from build123d import *

# Parameters (mm, degrees)
F1_DEPTH  = 25.4
F3_DEPTH  = 12.7
F4_R      = 19.05
F5_R      = 19.05
F6_R      = 20
F7_DEPTH  = 12.7
F8_R      = 21.5
F9_DEPTH  = 4.6
F10_R     = 33
F10_R_2   = 26.5
F11_DEPTH = 4
F12_W     = 3.69096
F12_H     = 9.525
F13_DEPTH = 8.7


with BuildPart() as f1:
    # F0 (on Top) → F1 (new body)
    with BuildSketch(Plane.XY):
        Polygon((22.73028, 39.37), (-22.73028, 39.37), (-45.46056, 0), (-22.73028, -39.37), (22.73028, -39.37), (45.46056, 0), align=None)
    extrude(amount=F1_DEPTH)

    # F2 (on face) → F3 (cut)
    with BuildSketch(Plane.XY.offset(25.4)):
        Polygon((21.26381, 36.83), (-21.26381, 36.83), (-42.527621, 0), (-21.26381, -36.83), (21.26381, -36.83), (42.527621, 0), align=None)
    extrude(amount=-F3_DEPTH, mode=Mode.SUBTRACT)

    # F4
    f4_edges = [f1.edges().sort_by_distance(p)[0] for p in [
        (21.26381, 36.83, 19.05),
        (-21.26381, 36.83, 19.05),
        (-42.527621, 0, 19.05),
        (42.527621, 0, 19.05),
        (21.26381, -36.83, 19.05),
        (-21.26381, -36.83, 19.05),
    ]]
    fillet(f4_edges, radius=F4_R)

    # F5
    f5_edges = [f1.edges().sort_by_distance(p)[0] for p in [
        (-22.73028, -39.37, 12.7),
        (22.73028, -39.37, 12.7),
        (45.46056, 0, 12.7),
        (-45.46056, 0, 12.7),
        (-22.73028, 39.37, 12.7),
        (22.73028, 39.37, 12.7),
    ]]
    fillet(f5_edges, radius=F5_R)

    # F6 (on face) → F7 (cut, through all)
    with BuildSketch(Plane(origin=(0, 0, 0), x_dir=(1, 0, 0), z_dir=(0, 0, -1))):
        Circle(F6_R)
    extrude(amount=-F7_DEPTH, mode=Mode.SUBTRACT)

    # F8 (on face) → F9 (cut)
    with BuildSketch(Plane(origin=(0, 0, 0), x_dir=(1, 0, 0), z_dir=(0, 0, -1))):
        Circle(F8_R)
    extrude(amount=-F9_DEPTH, mode=Mode.SUBTRACT)

    # F10 (on face) → F11 (cut)
    with BuildSketch(Plane(origin=(0, 0, 0), x_dir=(1, 0, 0), z_dir=(0, 0, -1))):
        Circle(F10_R)
        Circle(F10_R_2, mode=Mode.SUBTRACT)
    extrude(amount=-F11_DEPTH, mode=Mode.SUBTRACT)

    # F12 (on face) → F13 (cut, through all)
    with BuildSketch(Plane(origin=(0, 0, 4), x_dir=(1, 0, 0), z_dir=(0, 0, -1))):
        with Locations((29.75, 4.7625)):
            Rectangle(F12_W, F12_H)
        with Locations((29.75, -4.7625)):
            Rectangle(F12_W, F12_H)
    extrude(amount=-F13_DEPTH, mode=Mode.SUBTRACT)


solid = f1.part
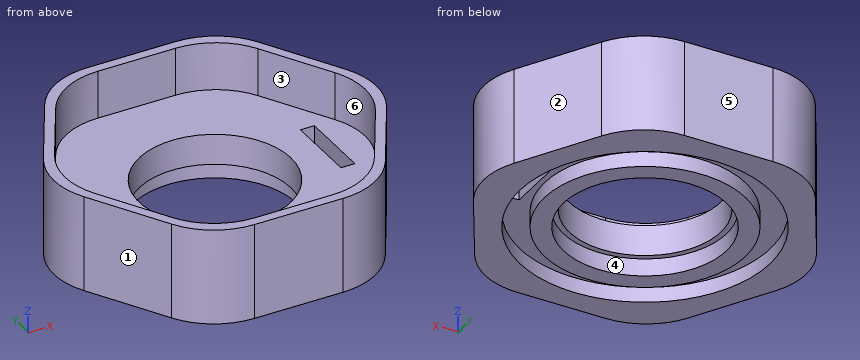
Read the model definition and answer for the solid it produces. Units are mm, in the model's axes. Face numbers are marked on the shaded views. A direction names the side the tool comes from. Coordinates: 2 decimals unless noted, no trailing zeros. Loops run counter-clockwise (first coordinate to the right, second up) from the corner with the lowest first, then second, coordinate; pieces in that order, holes last. Notation, with made-up numbers: (-2, 8) -> (50, 8) arc R9 cw to (50, 16) -> close; hole circle Ø2 at (57, -21). An arc over 180 degrees is marked (long way). Answer in a Markdown table with one row per item.
Item 1: For the marked faces 4, 5 and 6, determine the directions among +Z, -Z, +X, -X, +Y, -Y from which every point of the face is accessible in a straight line to the end or side of a thin tool.
Returned:
| item | result |
|---|---|
| face 4 | -Z |
| face 5 | +Z, -Z, +X, -X, +Y |
| face 6 | +Z |
Item 2: Each of these flat-tipped pins is pushed along its axis until it touches: P1, Ø7, axis at y = -2.5, z = 7, coming from the -X side; P2, Ø1.1, axis at x = 29.5, z = 7, coming from the -Y side; P3, Ø1.5, axis at x = -26.5, y = 31.5, coming from the -Z side; P4, Ø12, axis at x = -26.5, z = 14.5, coming from the -Y side. Where does it stop, or does it pass through?
Returned:
| item | result |
|---|---|
| P1 | stops at x = -42.51 |
| P2 | stops at y = -28.6 |
| P3 | stops at z = 0 |
| P4 | stops at y = -37.23 |
Item 3: A cutting plane is placed at D-D on y = 8.5. Determine the outline of the cut face in (x, z), plus the area to 3 significant figures.
Returned:
| item | result |
|---|---|
| outline | (-40.51, 0) -> (-31.89, 0) -> (-31.89, 4) -> (-25.1, 4) -> (-25.1, 0) -> (-19.75, 0) -> (-19.75, 4.6) -> (-18.1, 4.6) -> (-18.1, 12.7) -> (-37.58, 12.7) -> (-37.58, 25.4) -> (-40.51, 25.4) -> close; (18.1, 4.6) -> (19.75, 4.6) -> (19.75, 0) -> (25.1, 0) -> (25.1, 4) -> (27.9, 4) -> (27.9, 12.7) -> (18.1, 12.7) -> close; (31.6, 4) -> (31.89, 4) -> (31.89, 0) -> (40.51, 0) -> (40.51, 25.4) -> (37.58, 25.4) -> (37.58, 12.7) -> (31.6, 12.7) -> close |
| area | 542 mm^2 |
Item 4: For a pull along X with two mould halves and no side action, classify the marked faces 1, 2 and 3 as released by +X, released by -X, zero draft, split by the parting line, or undercut.
Returned:
| item | result |
|---|---|
| face 1 | released by -X |
| face 2 | released by +X |
| face 3 | undercut |
Item 5: Straight lines are drawn through the part: line 1 along X through (y, z) = (0, 1.2); line 2 along Y through (x, z) = (0, 1.2); line 3 along X through (y, z) = (0, 7). For each, find the intervals that lie inside material, in ascending order. Write a range as [from, to].
Returned:
| item | result |
|---|---|
| line 1 | x = [-42.51, -33], [-26.5, -21.5], [21.5, 26.5], [33, 42.51] |
| line 2 | y = [-39.37, -33], [-26.5, -21.5], [21.5, 26.5], [33, 39.37] |
| line 3 | x = [-42.51, -20], [20, 27.9], [31.6, 42.51] |
Item 6: A cutting plane is placed at A-A on y = 0. Determine the outline of the cut face in (x, z).
Returned:
| item | result |
|---|---|
| outline | (-42.51, 0) -> (-33, 0) -> (-33, 4) -> (-26.5, 4) -> (-26.5, 0) -> (-21.5, 0) -> (-21.5, 4.6) -> (-20, 4.6) -> (-20, 12.7) -> (-39.58, 12.7) -> (-39.58, 25.4) -> (-42.51, 25.4) -> close; (20, 4.6) -> (21.5, 4.6) -> (21.5, 0) -> (26.5, 0) -> (26.5, 4) -> (27.9, 4) -> (27.9, 12.7) -> (20, 12.7) -> close; (31.6, 4) -> (33, 4) -> (33, 0) -> (42.51, 0) -> (42.51, 25.4) -> (39.58, 25.4) -> (39.58, 12.7) -> (31.6, 12.7) -> close |
Item 7: A cutting plane is placed at B-B on x = 0. Determine the outline of the cut face in (y, z), plus the area to 3 significant figures.
Returned:
| item | result |
|---|---|
| outline | (-39.37, 0) -> (-33, 0) -> (-33, 4) -> (-26.5, 4) -> (-26.5, 0) -> (-21.5, 0) -> (-21.5, 4.6) -> (-20, 4.6) -> (-20, 12.7) -> (-36.83, 12.7) -> (-36.83, 25.4) -> (-39.37, 25.4) -> close; (20, 4.6) -> (21.5, 4.6) -> (21.5, 0) -> (26.5, 0) -> (26.5, 4) -> (33, 4) -> (33, 0) -> (39.37, 0) -> (39.37, 25.4) -> (36.83, 25.4) -> (36.83, 12.7) -> (20, 12.7) -> close |
| area | 491 mm^2 |
Item 8: A cutting plane is placed at C-C on z = 22.5. Determine the outline of the cut face in (x, y) (3 decimals).
Returned:
| item | result |
|---|---|
| outline | (-39.961, -9.525) -> (-28.23, -29.845) arc R19.05 ccw to (-11.732, -39.37) -> (11.732, -39.37) arc R19.05 ccw to (28.23, -29.845) -> (39.961, -9.525) arc R19.05 ccw to (39.961, 9.525) -> (28.23, 29.845) arc R19.05 ccw to (11.732, 39.37) -> (-11.732, 39.37) arc R19.05 ccw to (-28.23, 29.845) -> (-39.961, 9.525) arc R19.05 ccw to start; hole (-37.028, -9.525) -> (-26.763, -27.305) arc R19.05 ccw to (-10.265, -36.83) -> (10.265, -36.83) arc R19.05 ccw to (26.763, -27.305) -> (37.028, -9.525) arc R19.05 ccw to (37.028, 9.525) -> (26.763, 27.305) arc R19.05 ccw to (10.265, 36.83) -> (-10.265, 36.83) arc R19.05 ccw to (-26.763, 27.305) -> (-37.028, 9.525) arc R19.05 ccw to start |
